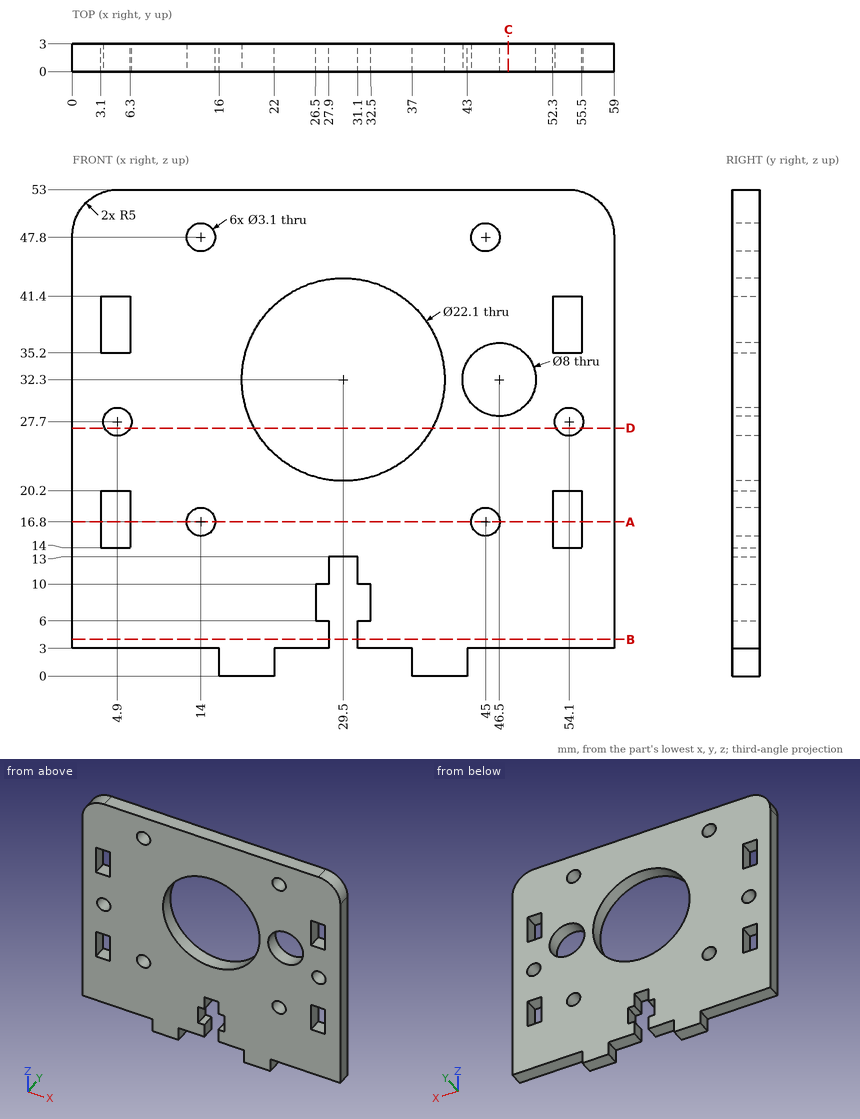
Study the drawing (mm; zero at the part's minimum x, y, z) and answer. Coordinates: 2 decimals unless noted, no trailing zeros. Order: outer loops, then holes, each group sorted by start corner. A loop starts at its lowest first (then second) coordinate and runs counter-clockwise, first axis right, second up. Notation, with made-up numbers: M -38,28 L 3,28 A28 ccw 3,54 Z; hole C 52.25,-7.75 d1. An arc over 180 degrees is marked long. Answer as a JSON object with one key per item and string values. Group by question number.
1. Section C-C on x = 47.5 is taken. Write down the section's boundary in (y, z).
2. Section D-D on z = 27 is taken. Write down the section's boundary in (x, y).
3. Straight lines are drawn through the part: line 1 (Z direction, x = 4.9, y = 1.1); line 2 (Z direction, x = 14, y = 2.1); line 3 (X direction, y = 2.35, z = 47.8). For each, find the intervals that lie inside material, in ascending order.
4. Section A-A on z = 16.8 is taken. Write down the section's boundary in (x, y).
5. A flat-ended cylindrical pin translates along its axis: P1, Ø1.5, axis at x = 32, y = 1, coming from the -Z side. Find the tip coordinate at first contact, or state that the pin passes through.
6. Section B-B on z = 4 is taken. Write down the section's boundary in (x, y).
Values follow:
{
 "1": {"outline": "M 0,3 L 3,3 L 3,28.43 L 0,28.43 Z; M 0,36.17 L 3,36.17 L 3,53 L 0,53 Z"},
 "2": {"outline": "M 0,0 L 3.52,0 L 3.52,3 L 0,3 Z; M 6.28,0 L 19.8,0 L 19.8,3 L 6.28,3 Z; M 39.2,0 L 52.72,0 L 52.72,3 L 39.2,3 Z; M 55.48,0 L 59,0 L 59,3 L 55.48,3 Z"},
 "3": {"line 1": "3 to 14, 20.2 to 26.15, 29.25 to 35.2, 41.4 to 53", "line 2": "3 to 15.25, 18.35 to 46.25, 49.35 to 53", "line 3": "0 to 12.45, 15.55 to 43.45, 46.55 to 59"},
 "4": {"outline": "M 0,0 L 3.1,0 L 3.1,3 L 0,3 Z; M 6.3,0 L 12.45,0 L 12.45,3 L 6.3,3 Z; M 15.55,0 L 43.45,0 L 43.45,3 L 15.55,3 Z; M 46.55,0 L 52.3,0 L 52.3,3 L 46.55,3 Z; M 55.5,0 L 59,0 L 59,3 L 55.5,3 Z"},
 "5": {"P1": "z = 3"},
 "6": {"outline": "M 0,0 L 27.9,0 L 27.9,3 L 0,3 Z; M 31.1,0 L 59,0 L 59,3 L 31.1,3 Z"}
}
